Geometry: final body of the model. Coordinates: model frame, mm. Give positions to 0.01 mm unless a question says otherwise; leave off trailing zeros. Loops run counter-clockwise (first coordinate to the right, second up) from the corner with the lowest first, then second, coordinate; pieces in that order, holes last. Notation, with made-up numbers: (66.25, 58.5) - (115.25, 58.5) arc R22 cw to (115.25, 72.5) - close; hole circle Ø8 at (46.5, -20.5). An arc over 180 degrees is marked (long way). Use one line per item in the form item = value.
```python
from build123d import *

# Parameters (mm, degrees)
F0_W          = 76.2
F0_H          = 609.6
F0_W_2        = 25.4
F0_H_2        = 152.4
F1_DEPTH      = 38.1
F1_DEPTH_BACK = 38.1
F2_W          = 25.4
F2_H          = 76.2
F3_DEPTH      = 101.6


with BuildPart() as f1:
    # F0 (on Right) → F1 (new body, two sides)
    with BuildSketch(Plane.YZ) as f1_sk:
        with Locations((0, -241.3)):
            Rectangle(F0_W, F0_H)
        with Locations((0, -165.1)):
            Rectangle(F0_W_2, F0_H_2, mode=Mode.SUBTRACT)
    extrude(amount=F1_DEPTH)
    extrude(f1_sk.sketch, amount=-F1_DEPTH_BACK)

    # F2 (on face) → F3 (cut)
    with BuildSketch(Plane.XZ.offset(38.1)):
        Rectangle(F2_W, F2_H)
        with Locations((0, -482.6)):
            Rectangle(F2_W, F2_H)
    extrude(amount=-F3_DEPTH, mode=Mode.SUBTRACT)


solid = f1.part
```
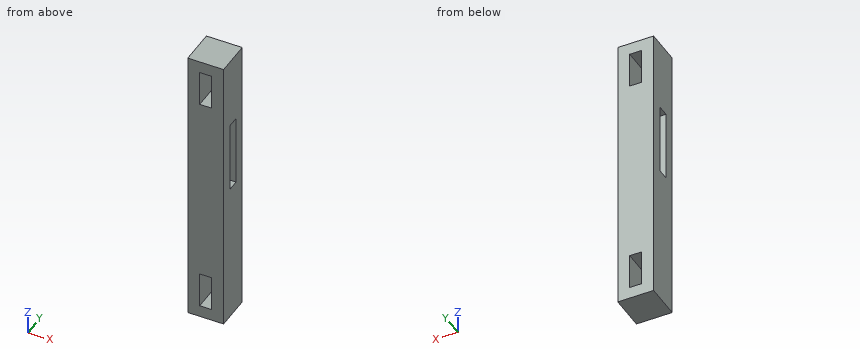
(1) Cut plane D-D (x = 30.5). Return the cut outline in (y, z), plus the area to 3 significant figures.
Solution:
outline = (-38.1, -546.1) - (38.1, -546.1) - (38.1, 63.5) - (-38.1, 63.5) - close; hole (-12.7, -241.3) - (12.7, -241.3) - (12.7, -88.9) - (-12.7, -88.9) - close
area = 42,600 mm2
(2) Material intervals for L1, parallel to Z at x = 1, y = 29.5; L2, parallel to Y at x = -1.5, z = -190.5, sorted ascending. Write a range as from..to.
Solution:
L1 = -546.1..-520.7, -444.5..-38.1, 38.1..63.5
L2 = -38.1..-12.7, 12.7..38.1
(3) Cut plane A-A (y = -0.5). Return the cut outline in (x, z), plus the area to 3 significant figures.
Solution:
outline = (-38.1, -546.1) - (38.1, -546.1) - (38.1, -241.3) - (-38.1, -241.3) - close; (-38.1, -88.9) - (38.1, -88.9) - (38.1, 63.5) - (-38.1, 63.5) - close; hole (-12.7, -520.7) - (12.7, -520.7) - (12.7, -444.5) - (-12.7, -444.5) - close; hole (-12.7, -38.1) - (12.7, -38.1) - (12.7, 38.1) - (-12.7, 38.1) - close
area = 31,000 mm2
(4) Cut plane B-B (z = -459). Return the cut outline in (x, y).
Solution:
outline = (-38.1, -38.1) - (-12.7, -38.1) - (-12.7, 38.1) - (-38.1, 38.1) - close; (12.7, -38.1) - (38.1, -38.1) - (38.1, 38.1) - (12.7, 38.1) - close
(5) Cut plane C-C (y = 23). Return the cut outline in (x, z).
Solution:
outline = (-38.1, -546.1) - (38.1, -546.1) - (38.1, 63.5) - (-38.1, 63.5) - close; hole (-12.7, -520.7) - (12.7, -520.7) - (12.7, -444.5) - (-12.7, -444.5) - close; hole (-12.7, -38.1) - (12.7, -38.1) - (12.7, 38.1) - (-12.7, 38.1) - close
